from build123d import *

# Parameters (mm, degrees)
SKETCH_1_W          = 15
SKETCH_1_H          = 15
SKETCH_1_W_2        = 13
SKETCH_1_H_2        = 13
EXTRUDE_1_DEPTH     = 240.3
SKETCH_2_R          = 1.45
CUT_EXTRUDE_1_DEPTH = 241.884495142
SKETCH_3_R          = 1.45
CUT_EXTRUDE_2_DEPTH = 241.884495142


with BuildPart() as part:
    # 草图1 → 凸台-拉伸1 (new body)
    with BuildSketch(Plane(origin=(0, 0, 0), x_dir=(0, 0, -1), z_dir=(1, 0, 0))):
        Rectangle(SKETCH_1_W, SKETCH_1_H)
        Rectangle(SKETCH_1_W_2, SKETCH_1_H_2, mode=Mode.SUBTRACT)
    extrude(amount=EXTRUDE_1_DEPTH)

    # 草图2 → 切除-拉伸1 (cut, through all)
    with BuildSketch(Plane(origin=(0, 7.5, 0), x_dir=(1, 0, 0), z_dir=(0, 1, 0))):
        with Locations(Location((5, 0, 0), (0, 0, 270))):
            Circle(SKETCH_2_R)
        with Locations(Location((15, 0, 0), (0, 0, 270))):
            Circle(SKETCH_2_R)
        with Locations(Location((36.30151519, 0, 0), (0, 0, 270))):
            Circle(SKETCH_2_R)
        with Locations(Location((56.30151519, 0, 0), (0, 0, 270))):
            Circle(SKETCH_2_R)
        with Locations(Location((99.30151519, 0, 0), (0, 0, 270))):
            Circle(SKETCH_2_R)
        with Locations(Location((221.30151519, 0, 0), (0, 0, 270))):
            Circle(SKETCH_2_R)
        with Locations(Location((231.30151519, 0, 0), (0, 0, 270))):
            Circle(SKETCH_2_R)
        with Locations(Location((131.30151519, 0, 0), (0, 0, 270))):
            Circle(SKETCH_2_R)
        with Locations(Location((161.30151519, 0, 0), (0, 0, 270))):
            Circle(SKETCH_2_R)
        with Locations(Location((191.30151519, 0, 0), (0, 0, 270))):
            Circle(SKETCH_2_R)
    extrude(amount=-CUT_EXTRUDE_1_DEPTH, mode=Mode.SUBTRACT)

    # 草图3 → 切除-拉伸2 (cut, through all)
    with BuildSketch(Plane.XY.offset(7.5)):
        with Locations((61.30151519, 0)):
            Circle(SKETCH_3_R)
        with Locations((226.30151519, 0)):
            Circle(SKETCH_3_R)
        with Locations((94.30151519, 0)):
            Circle(SKETCH_3_R)
    extrude(amount=-CUT_EXTRUDE_2_DEPTH, mode=Mode.SUBTRACT)


solid = part.part
Input: part model. Units: mm. Frame: model coordinates. A direction names the side the tool comes from. Coordinates: 2 decimals unless noted, no trailing zeros. Loops run counter-clockwise (first coordinate to the right, second up) from the corner with the lowest first, then second, coordinate; pieces in that order, holes last.
Q1. Cut plane B-B (z = 4.25). Output: boundary loops of the cut face in (x, y).
Q2. Draft query along Y for faces 3 (the face through (118, -7.5, 0)), 4 (the face through (118, 6.5, 0)), 5 (the face through (118, 7.5, 0)). Return one class per face: +Y half, -Y half, draft (parallel to the pull), parting line (faces both ways), or undercut.
Q3. Material intervals for line 1 (Y direction, x = 25, z = 5.25), sorted ascending.
Q4. Cut plane A-A (x = 138.5). Output: boundary loops of the cut face in (y, z), then the cut area to 3 significant figures.
Q5. Set-up query: faces 1 (the face through (118, -6.5, 0)), 2 (the face through (118, 0, -7.5)). Return all of +Z, -Z, +X, -X, +Y, -Y with unobstructed straight access to the full face (end or side cutting, diameter ignored); none if empty.
Working result:
1. outline: (0, -7.5) - (240.3, -7.5) - (240.3, -6.5) - (0, -6.5) - close; (0, 6.5) - (240.3, 6.5) - (240.3, 7.5) - (0, 7.5) - close
2. face 3: -Y half
2. face 4: undercut
2. face 5: +Y half
3. line 1: y = -7.5 to -6.5, 6.5 to 7.5
4. outline: (-7.5, -7.5) - (7.5, -7.5) - (7.5, 7.5) - (-7.5, 7.5) - close; hole (-6.5, -6.5) - (6.5, -6.5) - (6.5, 6.5) - (-6.5, 6.5) - close
4. area: 56.0 mm2
5. face 1: +X, -X
5. face 2: -Z, +X, -X, +Y, -Y
